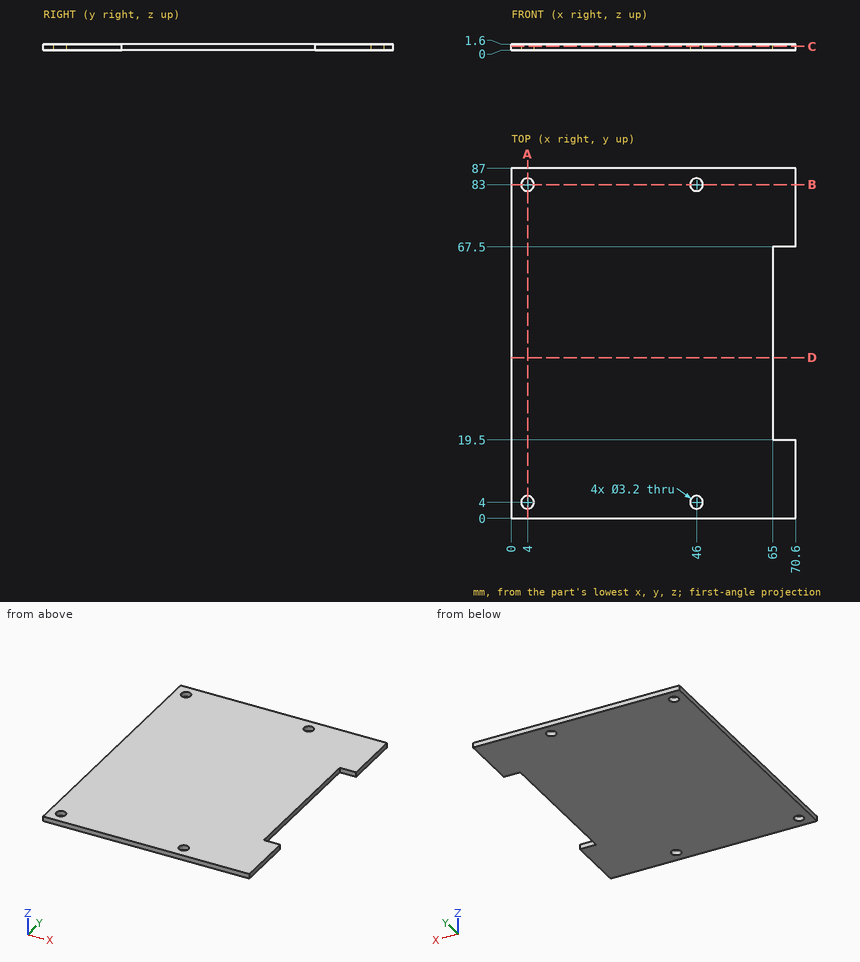
Check sheet for the drawn part. Datum: minimum x, y, z corner. Units: mm. Give positions to 0.01 mm unless a question says otherwise; leave off trailing zeros. Order: outer loops, then holes, each group sorted by start corner. A loop starts at its lowest first (then second) coordinate and runs counter-clockwise, first axis right, second up. Notation, with made-up numbers: (-35.75, 59.5) -> (0.25, 59.5) arc R17 cw to (0.25, 69.5) -> close; hole circle Ø8 at (53, 69.25). An arc over 180 degrees is marked (long way). Answer as CSV lines item,"result".
Q1. Sectioned sample at A-A on x = 4. Record the cut outline in (y, z), plus the area to 3 significant figures.
Solutions:
outline,"(0, 0) -> (2.4, 0) -> (2.4, 1.6) -> (0, 1.6) -> close; (5.6, 0) -> (81.4, 0) -> (81.4, 1.6) -> (5.6, 1.6) -> close; (84.6, 0) -> (87, 0) -> (87, 1.6) -> (84.6, 1.6) -> close"
area,"129 mm²"
Q2. Sectioned sample at C-C on z = 1. Record the cut outline in (x, y).
Solutions:
outline,"(0, 0) -> (70.6, 0) -> (70.6, 19.5) -> (65, 19.5) -> (65, 67.5) -> (70.6, 67.5) -> (70.6, 87) -> (0, 87) -> close; hole circle Ø3.2 at (4, 4); hole circle Ø3.2 at (4, 83); hole circle Ø3.2 at (46, 4); hole circle Ø3.2 at (46, 83)"
Q3. Sectioned sample at B-B on y = 83. Record the cut outline in (x, z).
Solutions:
outline,"(0, 0) -> (2.4, 0) -> (2.4, 1.6) -> (0, 1.6) -> close; (5.6, 0) -> (44.4, 0) -> (44.4, 1.6) -> (5.6, 1.6) -> close; (47.6, 0) -> (70.6, 0) -> (70.6, 1.6) -> (47.6, 1.6) -> close"
Q4. Scan lines: probe 1 along Y at (x, z) = (46, 1.05); probe 2 along X at (y, z) = (83, 0.7); probe 3 along Y at (x, z) = (67.5, 1.4). Record each from-to range of solid material in increasing order.
Solutions:
probe 1,"y = 0 to 2.4, 5.6 to 81.4, 84.6 to 87"
probe 2,"x = 0 to 2.4, 5.6 to 44.4, 47.6 to 70.6"
probe 3,"y = 0 to 19.5, 67.5 to 87"
Q5. Depth check by flat-ended pin: pin 1 (3 mm diameter, centred on x = 46, y = 83, fed in from -Z); pin 2 (0.8 mm diameter, centred on y = 34.5, z = 1, fed in from +X). Enter the tip coordinate at first touch or a pass-through.
Solutions:
pin 1,"passes through"
pin 2,"stops at x = 65"
Q6. Sectioned sample at D-D on y = 40. Record the cut outline in (x, z).
Solutions:
outline,"(0, 0) -> (65, 0) -> (65, 1.6) -> (0, 1.6) -> close"
